Answer from the drawing. Dimensions are ordinates in mm from the lowest x, y and z of the part. A direction names the side the tool comes from. Coordinates: 2 decimals unless noted, no trailing zeros. Write each loop counter-clockwise with the first axis right and the second up, starting at its lowest first coordinate (ties: lowest second). Pieces come first, ordered by that corner, then holes. Notation, with made-up numbers: (11, 9) -> (34, 9) arc R20 ccw to (34, 15) -> close; hole circle Ø5 at (69.5, 63.25). An arc over 180 degrees is marked (long way). Use CSV: the item, a comma, the result in double quotes.
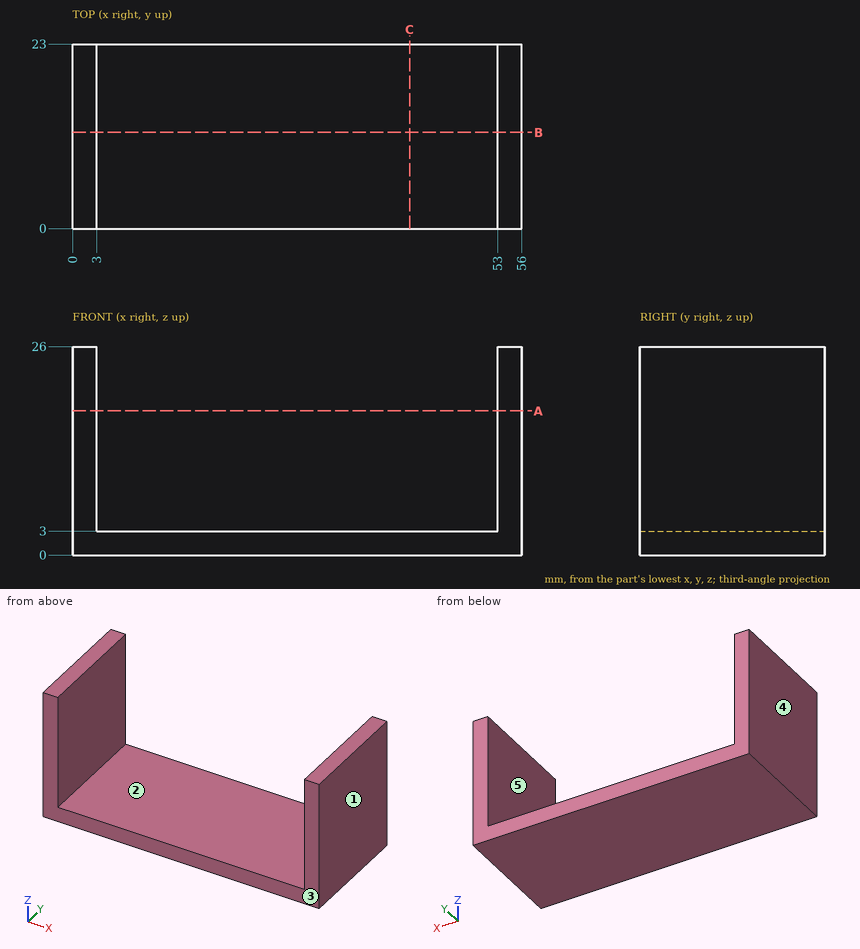
1. A cutting plane is placed at B-B (y = 12). Give the vertices of the cut face in (x, z), and give its area (3 significant figures).
Solutions:
outline,"(0, 0) -> (56, 0) -> (56, 26) -> (53, 26) -> (53, 3) -> (3, 3) -> (3, 26) -> (0, 26) -> close"
area,"306 mm^2"
2. A cutting plane is placed at A-A (z = 18). Give the vertices of the cut face in (x, y).
Solutions:
outline,"(0, 0) -> (3, 0) -> (3, 23) -> (0, 23) -> close; (53, 0) -> (56, 0) -> (56, 23) -> (53, 23) -> close"
3. A cutting plane is placed at C-C (x = 42). Give the vertices of the cut face in (y, z).
Solutions:
outline,"(0, 0) -> (23, 0) -> (23, 3) -> (0, 3) -> close"
4. For a pull along X with two mould halves and no side action, classify the marked faces 1, 2 and 3 as pulls with the +X half, pulls with the -X half, needs draft (parallel to the pull), parting line crosses it, or undercut.
Solutions:
face 1,"pulls with the +X half"
face 2,"undercut"
face 3,"needs draft"
5. A tool of negligible diameter and unlimited length cuts with its end or side. For the marked faces 4 and 5, from which of +Z, -Z, +X, -X, +Y, -Y can it reach the whole face along a straight path? Write none if from no direction.
Solutions:
face 4,"+Z, -Z, -X, +Y, -Y"
face 5,"+Z, +Y, -Y"
6. Each of these flat-tipped pins is pushed along its axis until it touches: pin 1 Ø10 at (x, z) = (48.5, 21.5) entering from -Y; pin 2 Ø6 at (x, y) = (34.5, 9.5) entering from +Z. Where does it stop, or does it pass through?
Solutions:
pin 1,"stops at y = 0"
pin 2,"stops at z = 3"
7. Find the intervals of material crossed by line 1 along X through (y, z) = (7, 23); line 2 along Z through (x, y) = (26, 5.25), in increasing order.
Solutions:
line 1,"x = 0 to 3, 53 to 56"
line 2,"z = 0 to 3"
